```python
from build123d import *

# Parameters (mm, degrees)
F0_R     = 2.5
F1_DEPTH = 115
F0_R_2   = 10
F2_DEPTH = 5
F3_R     = 1
F4_DEPTH = 5


with BuildPart() as f1:
    # F0 (on Top) → F1 (new body)
    with BuildSketch(Plane.XY):
        Circle(F0_R)
    extrude(amount=F1_DEPTH)

    # F0 (on Top) → F2 (join)
    with BuildSketch(Plane.XY):
        Circle(F0_R_2)
        Circle(F0_R, mode=Mode.SUBTRACT)
    extrude(amount=F2_DEPTH)

    # F3 (on Front) → F4 (cut, symmetric)
    with BuildSketch(Plane.XZ):
        with Locations((0, 111.190595)):
            Circle(F3_R)
    extrude(amount=F4_DEPTH, both=True, mode=Mode.SUBTRACT)


solid = f1.part
```
Here's how the part is built. I have some questions about the finished solid (model axes, mm). A direction names the side the tool comes from. Round coordinates to 2 decimals unless told otherwise and drop trailing zeros. Order: outer loops, then holes, each group sorted by start corner. A loop starts at its lowest first (then second) coordinate and runs counter-clockwise, first axis right, second up. Notation, with made-up numbers: M -32.75,-29 L -13.75,-29 A20 cw -13.75,-18 Z; hole C 84.25,31 d1. An arc over 180 degrees is marked long. Answer in a Markdown table with one row per item.
Item 1: I'm going to push flat-ended pins straight in: pin 1 (1 mm diameter, centred on x = 3.5, z = 23.5, fed in from -Y); pin 2 (10 mm diameter, centred on x = -4, y = 6.5, fed in from +Z); pin 3 (10 mm diameter, centred on y = 1, z = 18, fed in from +X); pin 4 (2.5 mm diameter, centred on x = 0, z = 111.19, fed in from +Y). Where does each tip first touch, or does it pass through?
A:
| item | result |
|---|---|
| pin 1 | passes through |
| pin 2 | stops at z = 5 |
| pin 3 | stops at x = 2.5 |
| pin 4 | stops at y = 2.5 |
Item 2: Imagine slicing it at C-C, the plane z = 35. Write out the boundary of the cut face in (x, y), and give its area (3 significant figures).
A:
| item | result |
|---|---|
| outline | C 0,0 d5 |
| area | 19.6 mm2 |
Item 3: Imagine slicing it at D-D, the plane x = 6.75. Write out the boundary of the cut face in (y, z), and give its area (3 significant figures).
A:
| item | result |
|---|---|
| outline | M -7.38,0 L 7.38,0 L 7.38,5 L -7.38,5 Z |
| area | 73.8 mm2 |
Item 4: Imagine slicing it at A-A, the plane x = 0. Write out the boundary of the cut face in (y, z).
A:
| item | result |
|---|---|
| outline | M -10,0 L 10,0 L 10,5 L 2.5,5 L 2.5,110.19 L -2.5,110.19 L -2.5,5 L -10,5 Z; M -2.5,112.19 L 2.5,112.19 L 2.5,115 L -2.5,115 Z |
Item 5: For faces 4 (the face through (-0.54, -2.44, 59.23)), 5 (the face through (0, 0, 0)), which set-ups out of +Z, -Z, +X, -X, +Y, -Y let a thin tool reach every point of the face, with its end or its side?
A:
| item | result |
|---|---|
| face 4 | +Z |
| face 5 | -Z, +X, -X, +Y, -Y |
Item 6: Thinking about a two-plate mould opening in X: for faces 1 (the face through (-2.17, -9.76, 2.46)), 2 (the face through (2, -2, 5)), 3 (the face through (-0.13, -0.035, 112.182)), which applies, +X half, -X half, draft (parallel to the pull), parting line (faces both ways), or undercut?
A:
| item | result |
|---|---|
| face 1 | parting line |
| face 2 | draft |
| face 3 | undercut |
Item 7: If I drill on L1, parallel to Z at x = 0, y = 0.55; L2, parallel to Z at x = -7.5, y = -4.5; L3, parallel to X at y = -2.25, z = 84, over which ranges is the centre line in solid material (lowest first)? Write a range as from..to.
A:
| item | result |
|---|---|
| L1 | z = 0..110.19, 112.19..115 |
| L2 | z = 0..5 |
| L3 | x = -1.09..1.09 |
Item 8: Imagine slicing it at B-B, the plane y = 0. Write out the boundary of the cut face in (x, z).
A:
| item | result |
|---|---|
| outline | M -10,0 L 10,0 L 10,5 L 2.5,5 L 2.5,115 L -2.5,115 L -2.5,5 L -10,5 Z; hole C 0,111.19 d2 |
